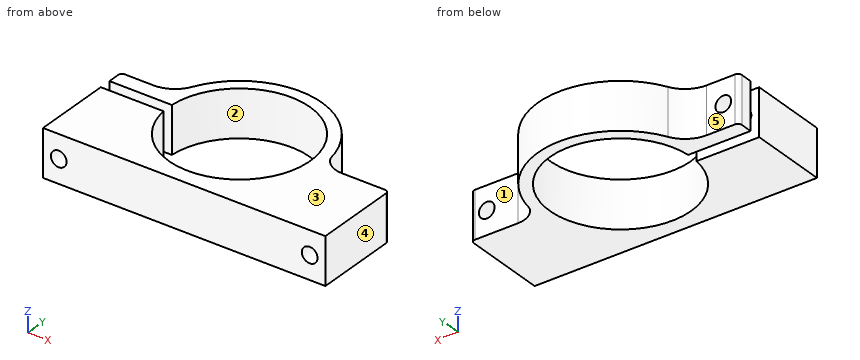
from build123d import *

# Parameters (mm, degrees)
BOSS_EXTRU_1_DEPTH      = 12
ESQUISSE2_R             = 2
ENL_V_MAT_EXTRU_2_DEPTH = 85.717176535
ESQUISSE2_4_R           = 2
ENL_V_MAT_EXTRU_3_DEPTH = 32
CONG_1_R                = 1


with BuildPart() as part:
    # Esquisse1 → Boss.-Extru.1 (new body)
    with BuildSketch(Plane.XY):
        with BuildLine():
            Line((0, 0), (72, 0))
            Line((72, 0), (72, 22))
            Line((72, 22), (60, 22))
            ThreePointArc((60, 22), (56.833671471, 22.903494958), (54.620930228, 25.341878785))
            ThreePointArc((54.620930228, 25.341878785), (36.966721004, 42.773175617), (15.016177647, 31.210526316))
            ThreePointArc((15.016177647, 31.210526316), (12.249643941, 28.139141071), (8.27604687, 27))
            Line((8.27604687, 27), (0, 27))
            Line((0, 27), (0, 23))
            Line((0, 23), (15.916343064, 23))
            ThreePointArc((15.916343064, 23), (51.881549416, 22.50174657), (16, 20))
            Line((16, 20), (0, 20))
            Line((0, 20), (0, 0))
        make_face()
    extrude(amount=BOSS_EXTRU_1_DEPTH)

    # Esquisse2 → Enl_v. mat.-Extru.2 (cut, through all)
    with BuildSketch(Plane(origin=(0, 0, 0), x_dir=(-1, 0, 0), z_dir=(0, -1, 0))):
        with Locations(Location((-4, -6, 0), (0, 0, 90))):
            Circle(ESQUISSE2_R)
    extrude(amount=-ENL_V_MAT_EXTRU_2_DEPTH, mode=Mode.SUBTRACT)

    # Esquisse2_4 → Enl_v. mat.-Extru.3 (cut)
    with BuildSketch(Plane(origin=(0, 0, 0), x_dir=(-1, 0, 0), z_dir=(0, -1, 0))):
        with Locations(Location((-4, -6, 0), (0, 0, 90))):
            Circle(ESQUISSE2_4_R)
        with Locations(Location((-68, -6, 0), (0, 0, 90))):
            Circle(ESQUISSE2_4_R)
    extrude(amount=-ENL_V_MAT_EXTRU_3_DEPTH, mode=Mode.SUBTRACT)

    # Cong_1
    cong_1_edges = [part.edges().sort_by_distance(p)[0] for p in [
        (72, 22, 6),
        (0, 27, 6),
    ]]
    fillet(cong_1_edges, radius=CONG_1_R)


solid = part.part
CAD build for the part. Positions are in the model's coordinates, mm. Face numbers are marked on the shaded views. A direction names the side the tool comes from. Round coordinates to 2 decimals unless told otherwise and drop trailing zeros. Write each loop counter-clockwise with the first axis right and the second up, starting at its lowest first coordinate (ties: lowest second). Pieces come first, ordered by that corner, then holes. Notation, with made-up numbers: (51.25, 37.25) -> (56.25, 37.25) arc R31 ccw to (56.25, 76.25) -> close; hole circle Ø9 at (77, -11). An arc over 180 degrees is marked (long way). Answer as a JSON object with one key per item and string values.
(1) Which spindle directions (+Z, -Z, +X, -X, +Y, -Y) get a long thin tool onto all of the face, cutting with end or side? Do the marked faces 4 and 5. Say none if no direction does.
Reported:
{"face 4": "+Z, -Z, +X, +Y, -Y", "face 5": "+Z, -Z, -X, +Y"}
(2) Band-saw the part on D-D, the plane x = 4. List the corners of the cut face in (y, z).
Reported:
{"outline": "(0, 0) -> (20, 0) -> (20, 4) -> (0, 4) -> close; (0, 8) -> (20, 8) -> (20, 12) -> (0, 12) -> close; (23, 0) -> (27, 0) -> (27, 4) -> (23, 4) -> close; (23, 8) -> (27, 8) -> (27, 12) -> (23, 12) -> close"}
(3) Probe probe 1 along X at (y, z) = (25.35, 6); probe 2 along X at (y, z) = (25.25, 6); probe 3 along Y at (x, z) = (66.5, 0.75). List the from-to ranges inside material, lowest first. Write a range as [from, to].
Reported:
{"probe 1": "x = [0, 2], [6, 16.2], [51.57, 54.62]", "probe 2": "x = [0, 2], [6, 16.18], [51.59, 54.67]", "probe 3": "y = [0, 22]"}
(4) Band-saw the part on C-C, the plane y = 10.5. List the corners of the cut face in (x, z).
Reported:
{"outline": "(0, 0) -> (20.04, 0) -> (20.04, 12) -> (0, 12) -> close; (47.74, 0) -> (72, 0) -> (72, 12) -> (47.74, 12) -> close; hole circle Ø4 at (4, 6); hole circle Ø4 at (68, 6)"}
(5) Two-plate mould, pull along Y, no slides. Class the marked faces 1, 2 and 3: +Y half, -Y half, draft (parallel to the pull), parting line (faces both ways), or undercut.
Reported:
{"face 1": "+Y half", "face 2": "undercut", "face 3": "draft"}
(6) Band-saw the part on B-B, the plane x = 68. List the corners of the cut face in (y, z).
Reported:
{"outline": "(0, 0) -> (22, 0) -> (22, 4) -> (0, 4) -> close; (0, 8) -> (22, 8) -> (22, 12) -> (0, 12) -> close"}
(7) Band-saw the part on A-A, the plane z = 6. List the corners of the cut face in (x, y), then the cut area to 3 significant figures.
Reported:
{"outline": "(0, 0) -> (2, 0) -> (2, 20) -> (0, 20) -> close; (0, 23) -> (2, 23) -> (2, 27) -> (1, 27) arc R1 ccw to (0, 26) -> close; (6, 0) -> (66, 0) -> (66, 22) -> (60, 22) arc R6 cw to (54.62, 25.34) arc R21 ccw to (15.02, 31.21) arc R7.5 cw to (8.28, 27) -> (6, 27) -> (6, 23) -> (15.92, 23) arc R18 cw (long way) to (16, 20) -> (6, 20) -> close; (70, 0) -> (72, 0) -> (72, 21) arc R1 ccw to (71, 22) -> (70, 22) -> close", "area": "1,100 mm^2"}
(8) Pin check, flat tips, straight feed: P1, Ø4, axis at x = 52, z = 8, coming from the +Y side; P2, Ø3.5, axis at x = 5.5, z = 3, coming from the +Y side; P3, Ø3, axis at x = 52, z = 1.5, coming from the +Y side. Stop position of each tip, or through.
Reported:
{"P1": "stops at y = 35.47", "P2": "stops at y = 27", "P3": "stops at y = 34.85"}
